CAD build for the part. Positions are in the model's coordinates, mm. A direction names the side the tool comes from. Coordinates: 2 decimals unless noted, no trailing zeros. Write each loop counter-clockwise with the first axis right and the second up, starting at its lowest first coordinate (ties: lowest second). Pieces come first, ordered by that corner, then holes. Notation, with made-up numbers: (-34, -21) -> (-29, -21) arc R11 cw to (-29, -10) -> close; hole circle Ø2 at (43, 43). An arc over 180 degrees is marked (long way). Answer as CSV lines item,"result".
```python
from build123d import *

# Parameters (mm, degrees)
F1_DEPTH = 12
F2_R     = 3
F3_DEPTH = 12.001
F4_R     = 2.5
F5_DEPTH = 4
F6_R     = 1.5
F7_DEPTH = 5


with BuildPart() as f1:
    # F0 (on Top) → F1 (new body)
    with BuildSketch(Plane.XY):
        Polygon((25.683252, 22.42391), (-19.316748, 22.42391), (-19.316748, 10.42391), (55.683252, 10.42391), (55.683252, 12.92391), align=None)
    extrude(amount=F1_DEPTH)

    # F2 (on face) → F3 (cut, through all)
    with BuildSketch(Plane(origin=(0, 22.42391, 0), x_dir=(-1, 0, 0), z_dir=(0, 1, 0))):
        with Locations((-18.683252, 6)):
            Circle(F2_R)
    extrude(amount=-F3_DEPTH, mode=Mode.SUBTRACT)

    # F4 (on face) → F5 (cut)
    with BuildSketch(Plane.XZ.offset(-10.42391)):
        with Locations((-11.316748, 6)):
            Circle(F4_R)
    extrude(amount=-F5_DEPTH, mode=Mode.SUBTRACT)

    # F6 (on face) → F7 (cut)
    with BuildSketch(Plane(origin=(0, 22.42391, 0), x_dir=(-1, 0, 0), z_dir=(0, 1, 0))):
        with Locations((-10.683252, 6)):
            Circle(F6_R)
    extrude(amount=-F7_DEPTH, mode=Mode.SUBTRACT)


solid = f1.part
```
Item 1: Saw through at C-C on x = 39. Give the cut face in (y, z).
Answer below:
outline,"(10.42, 0) -> (18.21, 0) -> (18.21, 12) -> (10.42, 12) -> close"
Item 2: Saw through at A-A on z = 6. Give the cut face in (x, y).
Answer below:
outline,"(-19.32, 10.42) -> (-13.82, 10.42) -> (-13.82, 14.42) -> (-8.82, 14.42) -> (-8.82, 10.42) -> (15.68, 10.42) -> (15.68, 22.42) -> (12.18, 22.42) -> (12.18, 17.42) -> (9.18, 17.42) -> (9.18, 22.42) -> (-19.32, 22.42) -> close; (21.68, 10.42) -> (55.68, 10.42) -> (55.68, 12.92) -> (25.68, 22.42) -> (21.68, 22.42) -> close"
Item 3: Two-plate mould, pull along X, no slides. Class faces 1 (the flat face through (55.683, 12, 6)), 2 (the cylindrical face through (21.68, 16.51, 6.13)), 3 (the flat face through (3, 22.424, 6)): pulls with the +X half, pulls with the -X half, needs draft (parallel to the pull), parting line crosses it, or undercut.
Answer below:
face 1,"pulls with the +X half"
face 2,"undercut"
face 3,"needs draft"
Item 4: 3-axis set-ups, long thin cutter, end or side, ignore diameter. For faces 4 (the cylindrical face through (-8.93, 12.4, 6.75)), 5 (the flat face through (11, 17.424, 6)), 6 (the flat face through (18, 10.424, 2)): which of +Z, -Z, +X, -X, +Y, -Y reach the whole face in a straight line?
Answer below:
face 4,"-Y"
face 5,"+Y"
face 6,"+Z, -Z, +X, -X, -Y"
Item 5: Flat gauge pin, fed straight in: pin 1 (7 mm diameter, centred on x = 18.68, z = 6, fed in from +Y). Where does the tip first touch, or does it go through?
Answer below:
pin 1,"stops at y = 22.42"
Item 6: Wall check: line 1 (Z direction, x = 18.5, y = 21.75); line 2 (Y direction, x = 27, z = 5.5); line 3 (Y direction, x = 41.5, z = 6.75). Give the ranges that are in metal, low to high. Write a range as from..to.
Answer below:
line 1,"z = 0..3.01, 8.99..12"
line 2,"y = 10.42..22.01"
line 3,"y = 10.42..17.42"
Item 7: Saw through at B-B on z = 11. Give the cut face in (x, y).
Answer below:
outline,"(-19.32, 10.42) -> (55.68, 10.42) -> (55.68, 12.92) -> (25.68, 22.42) -> (-19.32, 22.42) -> close"
